from build123d import *

# Parameters (mm, degrees)
F1_DEPTH = 2700
F2_W     = 175
F2_H     = 20
F3_DEPTH = 46.001
F4_W     = 29.575
F4_H     = 90
F4_W_2   = 9
F5_DEPTH = 46.001
F6_W     = 74
F6_H     = 62
F7_DEPTH = 46.001


with BuildPart() as f1:
    # F0 (on Top) → F1 (new body)
    with BuildSketch(Plane.XY):
        with BuildLine():
            Line((-127.6665818456, 21), (-127.6665818456, 0))
            Line((-127.6665818456, 0), (-121.6665818456, 0))
            Line((-121.6665818456, 0), (-121.6665818456, 15))
            ThreePointArc((-121.6665818456, 15), (-119.0305428763, 21.3639610307), (-112.6665818456, 24))
            Line((-112.6665818456, 24), (-12.6665818456, 24))
            Line((-12.6665818456, 24), (-12.6665818456, 30))
            Line((-12.6665818456, 30), (-118.6665818456, 30))
            ThreePointArc((-118.6665818456, 30), (-125.0305428763, 27.3639610307), (-127.6665818456, 21))
        make_face()
        with BuildLine():
            Line((93.3334181544, 30), (-12.6665818456, 30))
            Line((-12.6665818456, 30), (-12.6665818456, 24))
            Line((-12.6665818456, 24), (87.3334181544, 24))
            ThreePointArc((87.3334181544, 24), (93.697379185, 21.3639610307), (96.3334181544, 15))
            Line((96.3334181544, 15), (96.3334181544, -7))
            ThreePointArc((96.3334181544, -7), (98.9694571237, -13.3639610307), (105.3334181544, -16))
            Line((105.3334181544, -16), (152.3334181544, -16))
            Line((152.3334181544, -16), (152.3334181544, -10))
            Line((152.3334181544, -10), (111.3334181544, -10))
            ThreePointArc((111.3334181544, -10), (104.9694571237, -7.3639610307), (102.3334181544, -1))
            Line((102.3334181544, -1), (102.3334181544, 21))
            ThreePointArc((102.3334181544, 21), (99.697379185, 27.3639610307), (93.3334181544, 30))
        make_face()
    extrude(amount=F1_DEPTH)

    # F2 (on face) → F3 (cut, through all)
    with BuildSketch(Plane(origin=(0, 30, 0), x_dir=(-1, 0, 0), z_dir=(0, 1, 0))):
        with Locations((40.1665818456, 2690)):
            Rectangle(F2_W, F2_H)
        Polygon((-47.3334181544, 0), (118.6665818456, 0), (127.6665818456, 0), (127.6665818456, 20), (-47.3334181544, 20), align=None)
    extrude(amount=-F3_DEPTH, mode=Mode.SUBTRACT)

    # F4 (on face) → F5 (cut, through all)
    with BuildSketch(Plane(origin=(0, 30, 0), x_dir=(-1, 0, 0), z_dir=(0, 1, 0))):
        with Locations((103.8790818456, 2452)):
            Rectangle(F4_W, F4_H)
        with Locations((123.1665818456, 2452)):
            Rectangle(F4_W_2, F4_H)
        with Locations((123.1665818456, 248)):
            Rectangle(F4_W_2, F4_H)
        with Locations((103.8790818456, 248)):
            Rectangle(F4_W, F4_H)
        with Locations((103.8790818456, 1078)):
            Rectangle(F4_W, F4_H)
        with Locations((123.1665818456, 1078)):
            Rectangle(F4_W_2, F4_H)
        with Locations((103.8790818456, 1622)):
            Rectangle(F4_W, F4_H)
        with Locations((123.1665818456, 1622)):
            Rectangle(F4_W_2, F4_H)
    extrude(amount=-F5_DEPTH, mode=Mode.SUBTRACT)

    # F6 (on face) → F7 (cut, through all)
    with BuildSketch(Plane(origin=(0, 30, 0), x_dir=(-1, 0, 0), z_dir=(0, 1, 0))):
        Polygon((-47.3334181544, 2680), (-47.3334181544, 2700), (-93.3334181544, 2700), (-93.3334181544, 2638), (-47.3334181544, 2638), align=None)
        with Locations((-130.3334181544, 2669)):
            Rectangle(F6_W, F6_H)
    extrude(amount=-F7_DEPTH, mode=Mode.SUBTRACT)


solid = f1.part
Design review of the part built by this model. Coordinates are the model's own, in mm. A direction names the side the tool comes from. Round coordinates to 2 decimals unless told otherwise and drop trailing zeros. Order: outer loops, then holes, each group sorted by start corner. A loop starts at its lowest first (then second) coordinate and runs counter-clockwise, first axis right, second up. Notation, with made-up numbers: M -18,35.25 L 37,35.25 A13 cw 37,57.25 Z; hole C 23.5,32 d2. An arc over 180 degrees is marked long. Answer as CSV lines item,"result". Start each with the question number.
1) Wall thickness on line 1 along X through (y, z) = (15, 611); line 2 along Y through (x, z) = (-114.5, 2081.5); line 3 along Y through (x, z) = (129, 1353.5): over which ranges is each line inside the solid? List them lowest first. Write a range as [from, to].
2) Add section B-B (x = -12). Give the boundary of the cut face in (y, z), then the cut area to 3 significant figures.
3) Add section A-A (z = 1757). Give the boundary of the cut face in (x, y), then the cut area to 3 significant figures.
4) Tool access review of faces 1 (the face through (132, -10, 1301)), 2 (the face through (100, 9, 2638)), 3 (the face through (-14, 24, 1321)): name each direction out of +Z, -Z, +X, -X, +Y, -Y from which nothing blocks a thin tool from reaching the whole face with its end or side.
5) For pin 1 Ø3 at (y, z) = (27.5, 1608) entering from -X; pin 2 Ø12 at (y, z) = (4.5, 2073.5) entering from +X; pin 3 Ø10 at (x, z) = (110.5, 1812.5) entering from +Y, all flat-tipped, find the tip position at first contact; note any pin that passes through.
Resolved:
1,line 1,"[-127.67, -121.67], [96.33, 102.33]"
1,line 2,"[23.81, 30]"
1,line 3,"[-16, -10]"
2,outline,"M 24,20 L 30,20 L 30,2680 L 24,2680 Z"
2,area,"16,000 mm^2"
3,outline,"M -127.67,0 L -121.67,0 L -121.67,15 A9 cw -112.67,24 L 87.33,24 A9 cw 96.33,15 L 96.33,-7 A9 ccw 105.33,-16 L 152.33,-16 L 152.33,-10 L 111.33,-10 A9 cw 102.33,-1 L 102.33,21 A9 ccw 93.33,30 L -118.67,30 A9 ccw -127.67,21 Z"
3,area,"2,060 mm^2"
4,face 1,"+Z, -Z, +X, +Y"
4,face 2,"+Z, +X, +Y, -Y"
4,face 3,"+Z, -Z, -Y"
5,pin 1,"x = -89.09"
5,pin 2,"x = 102.35"
5,pin 3,"y = -7.85"
